```python
from build123d import *

# Parameters (mm, degrees)
F0_R     = 28.575
F1_DEPTH = 40.2336
F2_R     = 10.16
F3_DEPTH = 15.7734
F4_R     = 3.302
F5_R     = 2.102171
F6_DEPTH = 25.4


with BuildPart() as f1:
    # F0 (on Top) → F1 (new body)
    with BuildSketch(Plane.XY):
        Circle(F0_R)
        with BuildLine():
            ThreePointArc((13.447765, -4.826), (-14.2875, 0), (13.447765, 4.826))
            Line((13.447765, 4.826), (18.5293, 4.826))
            Line((18.5293, 4.826), (18.5293, -4.826))
            Line((18.5293, -4.826), (13.447765, -4.826))
        make_face(mode=Mode.SUBTRACT)
    extrude(amount=F1_DEPTH)

    # F2 (on Top) → F3 (join)
    with BuildSketch(Plane.XY):
        with BuildLine():
            Line((5.042647, -28.126541), (57.336765, -18.751028))
            ThreePointArc((57.336765, -18.751028), (73.025, 0), (57.336765, 18.751028))
            Line((57.336765, 18.751028), (5.042647, 28.126541))
            ThreePointArc((5.042647, 28.126541), (28.575, 0), (5.042647, -28.126541))
        make_face()
        with Locations((53.975, 0)):
            Circle(F2_R, mode=Mode.SUBTRACT)
    extrude(amount=F3_DEPTH)

    # F4
    f4_edges = [f1.edges().sort_by_distance(p)[0] for p in [
        (-28.575, 0, 40.2336),
    ]]
    fillet(f4_edges, radius=F4_R)

    # F5 (on face) → F6 (join)
    with BuildSketch(Plane.XY.offset(40.2336)):
        with Locations((-6.10288, -20.530477)):
            Circle(F5_R)
    extrude(amount=F6_DEPTH)


solid = f1.part
```
Here's how the part is built. I have some questions about the finished solid (model axes, mm). A direction names the side the tool comes from. Give positions to 0.01 mm unless a question says otherwise; leave off trailing zeros. Write each loop counter-clockwise with the first axis right and the second up, starting at its lowest first coordinate (ties: lowest second). Pieces come first, ordered by that corner, then holes. Notation, with made-up numbers: M 86.25,82.5 L 90.25,82.5 A17 ccw 90.25,89.5 Z; hole C 68,88.5 d1. An arc over 180 degrees is marked long. Put each result on its own line as item: value. Start each with the question number.
Item 1: If we section it at A-A, the plane x = 0: Write out the boundary of the cut face in (y, z) (1 decimal), then the cut area to 3 significant figures.
Item 2: Thinking about a two-plate mould opening in X: for faces 1 (the cylindrical face through (73.02, -0.37, 7.78)), 2 (the flat face through (16, 4.826, 20)), 3 (the flat face through (39, 0, 15.773)), which applies, +X half, -X half, draft (parallel to the pull), parting line (faces both ways), or undercut?
Item 3: I need wall thicknesses on L1, parallel to X at y = 0, z = 23 (1 decimal); L2, parallel to Y at x = 0, z = 31 (1 decimal); L3, parallel to Z at x = 45, y = -14. Which ranges of each line are inside material? Lowest first, please. Write a range as from..to.
Item 4: On a 3-axis mill with a long thin cutter (end or side, diameter ignored), from which of +Z, -Z, +X, -X, +Y, -Y can I reach the whole of each face in a straight line? I mean faces 4 (the flat face through (31.558, 23.373, 7.776)), 5 (the cylindrical face through (-28.547, 1.256, 22.311)), 6 (the flat face through (16, -4.826, 20)). Say none if no direction works.
Item 5: If we section it at B-B, the plane y = 0: Write out the boundary of the cut face in (x, z) (1 decimal).
Item 6: Will these pins go through, and if not, where does the flat tip stop? pin 1 (12 mm diameter, centred on y = -8, z = 34, fed in from -X); pin 2 (1 mm diameter, centred on y = 5.5, z = 40, fed in from +X); pin 3 (8 mm diameter, centred on x = 4, z = 40.5, fed in from -Y); pin 4 (15 mm diameter, centred on x = -3, y = 5.5, fed in from +Z).
Item 7: If we section it at D-D, the plane z = 62: Write out the boundary of the cut face in (x, y).
Item 8: If we section it at C-C, the plane z = 39: Write out the boundary of the cut face in (x, y) (1 decimal).
Values:
1. outline: M -28.6,0 L -14.3,0 L -14.3,40.2 L -25.3,40.2 A3.3 ccw -28.6,36.9 Z; M 14.3,0 L 28.6,0 L 28.6,36.9 A3.3 ccw 25.3,40.2 L 14.3,40.2 Z
1. area: 1,140 mm²
2. face 1: +X half
2. face 2: undercut
2. face 3: draft
3. L1: -28.6..-14.3, 18.5..28.6
3. L2: -28.6..-14.3, 14.3..28.6
3. L3: 0..15.77
4. face 4: +Z, -Z, +X, +Y
4. face 5: +Z
4. face 6: +Z, -Z
5. outline: M -28.6,0 L -14.3,0 L -14.3,40.2 L -25.3,40.2 A3.3 ccw -28.6,36.9 Z; M 18.5,0 L 43.8,0 L 43.8,15.8 L 28.6,15.8 L 28.6,36.9 A3.3 ccw 25.3,40.2 L 18.5,40.2 Z; M 64.1,0 L 73,0 L 73,15.8 L 64.1,15.8 Z
6. pin 1: x = -28.5
6. pin 2: x = 26.8
6. pin 3: y = -28.51
6. pin 4: through
7. outline: C -6.1,-20.53 d4.2
8. outline: C 0,0 d55.7; hole M 13.4,-4.8 L 18.5,-4.8 L 18.5,4.8 L 13.4,4.8 A14.3 ccw long Z
